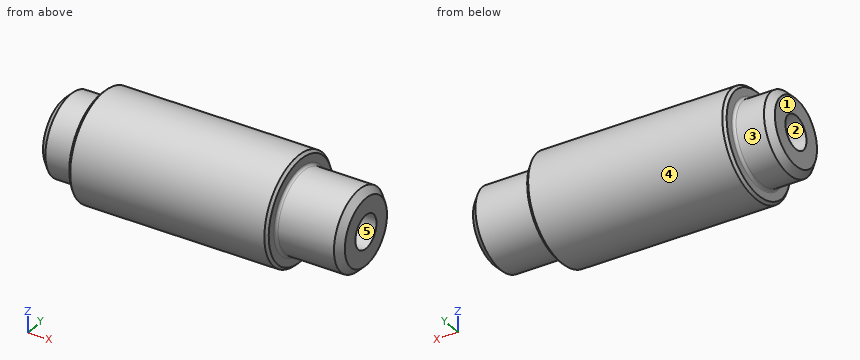
from build123d import *

# Parameters (mm, degrees)
TAPPED_HOLE1_D     = 2.5
TAPPED_HOLE1_DEPTH = 8.5
TAPPED_HOLE1_TIP   = 0.751075774
TAPPED_HOLE2_D     = 2.5
TAPPED_HOLE2_DEPTH = 8.5
TAPPED_HOLE2_TIP   = 0.751075774
CHAMFER1_SIZE      = 0.2
CHAMFER2_SIZE      = 0.2
CHAMFER3_SIZE      = 0.5
FILLET1_R          = 0.2
FILLET2_R          = 0.2


with BuildPart() as part:
    # Sketch1 → Revolve1 (revolve)
    with BuildSketch(Plane.XY, mode=Mode.PRIVATE) as revolve1_sk:
        Polygon((0, 0), (22.7, 0), (22.7, 3), (17.8, 3), (17.8, 4), (2.8, 4), (2.8, 3), (0, 3), align=None)
    revolve(revolve1_sk.sketch.rotate(Axis((0, 0, 0), (1, 0, 0)), 90), axis=Axis((0, 0, 0), (1, 0, 0)))

    # Tapped Hole1
    with Locations(Plane.ZY):
        with Locations((0, 0)):
            Hole(TAPPED_HOLE1_D / 2, depth=TAPPED_HOLE1_DEPTH)
            with Locations((0, 0, -(TAPPED_HOLE1_DEPTH + TAPPED_HOLE1_TIP / 2))):  # 118° drill point
                Cone(0, TAPPED_HOLE1_D / 2, TAPPED_HOLE1_TIP, mode=Mode.SUBTRACT)

    # Tapped Hole2
    with Locations(Plane(origin=(22.7, 0, 0), x_dir=(0, 0, -1), z_dir=(1, 0, 0))):
        with Locations((0, 0)):
            Hole(TAPPED_HOLE2_D / 2, depth=TAPPED_HOLE2_DEPTH)
            with Locations((0, 0, -(TAPPED_HOLE2_DEPTH + TAPPED_HOLE2_TIP / 2))):  # 118° drill point
                Cone(0, TAPPED_HOLE2_D / 2, TAPPED_HOLE2_TIP, mode=Mode.SUBTRACT)

    # Chamfer1
    chamfer1_edges = [part.edges().sort_by_distance(p)[0] for p in [
        (17.8, 0, -4),
    ]]
    chamfer(chamfer1_edges, length=CHAMFER1_SIZE)

    # Chamfer2
    chamfer2_edges = [part.edges().sort_by_distance(p)[0] for p in [
        (2.8, 0, -4),
    ]]
    chamfer(chamfer2_edges, length=CHAMFER2_SIZE)

    # Chamfer3
    chamfer3_edges = [part.edges().sort_by_distance(p)[0] for p in [
        (0, 0, -3),
        (22.7, 0, -3),
    ]]
    chamfer(chamfer3_edges, length=CHAMFER3_SIZE)

    # Fillet1
    fillet1_edges = [part.edges().sort_by_distance(p)[0] for p in [
        (2.8, 0, -3),
    ]]
    fillet(fillet1_edges, radius=FILLET1_R)

    # Fillet2
    fillet2_edges = [part.edges().sort_by_distance(p)[0] for p in [
        (17.8, 0, -3),
    ]]
    fillet(fillet2_edges, radius=FILLET2_R)


solid = part.part
Geometry check sheet. Reference: the model listing, model coordinates, mm. Face numbers are marked on the shaded views. A direction names the side the tool comes from. Give positions to 0.01 mm unless a question says otherwise; leave off trailing zeros. Loops run counter-clockwise (first coordinate to the right, second up) from the corner with the lowest first, then second, coordinate; pieces in that order, holes last. Notation, with made-up numbers: M -4,-9 L 10,-9 A6 ccw 10,-5 Z; hole C -37.75,74 d5. An arc over 180 degrees is marked long. Answer as a JSON object with one key per item and string values. Group by question number.
Item 1: Sectioned sample at B-B on x = 9.5. Record the boundary of the cut face in (y, z).
Item 2: Gauge pin test, flat ends, axial feed: pin 1 (2 mm diameter, centred on x = 12.5, z = 1, fed in from -Y); pin 2 (2 mm diameter, centred on y = 0, z = 0, fed in from +X); pin 3 (1.5 mm diameter, centred on x = 12, y = 2.5, fed in from -Z). Record the tip position at first contact, or that the pin passes through.
Item 3: Mould release check, pull along Z, two halves, no side actions. Record for the marked faces 1, 2 and 3: pulls with the +Z half, pulls with the -Z half, needs draft (parallel to the pull), parting line crosses it, or undercut.
Item 4: Access from +Z, -Z, +X, -X, +Y, -Y to the whole of each face (thin tool, end or side, straight path). Record for the marked faces 4 and 5.
Item 5: Sectioned sample at A-A on x = 16. Record the boundary of the cut face in (y, z).
Item 6: Sectioned sample at C-C on x = 18.75. Record the boundary of the cut face in (y, z).
Item 7: Material ranges on L1, parallel to Y at x = 20, z = 0; L2, parallel to X at y = 3.5, z = 0.5; L3, parallel to Y at x = 17.5, z = -1, recorded low to high.
Findings below:
{
 "1": {"outline": "C 0,0 d8"},
 "2": {"pin 1": "y = -4", "pin 2": "x = 14.05", "pin 3": "z = -3.6"},
 "3": {"face 1": "needs draft", "face 2": "undercut", "face 3": "parting line crosses it"},
 "4": {"face 4": "+X, -X", "face 5": "+X"},
 "5": {"outline": "C 0,0 d8; hole C 0,0 d2.5"},
 "6": {"outline": "C 0,0 d6; hole C 0,0 d2.5"},
 "7": {"L1": "-3 to -1.25, 1.25 to 3", "L2": "2.8 to 17.8", "L3": "-3.87 to -0.75, 0.75 to 3.87"}
}
